from build123d import *

# Parameters (mm, degrees)
ESBO_O1_W                  = 46
ESBO_O1_H                  = 40.25
ESBO_O1_R                  = 14
RESSALTO_EXTRUS_O1_DEPTH   = 5.3
ESBO_O2_W                  = 41.7
ESBO_O2_H                  = 40.25
ESBO_O2_R                  = 1.025
RESSALTO_EXTRUS_O2_DEPTH   = 3
ESBO_O3_W                  = 49
ESBO_O3_H                  = 41.7
RESSALTO_EXTRUS_O3_DEPTH   = 3
ESBO_O4_W                  = 41.7
ESBO_O4_H                  = 43.25
RESSALTO_EXTRUS_O4_DEPTH   = 3
ESBO_O5_W                  = 52
ESBO_O5_H                  = 41.7
RESSALTO_EXTRUS_O5_DEPTH   = 3
CORTE_EXTRUS_O1_DEPTH      = 66.274234005
CORTE_EXTRUS_O1_DEPTH_BACK = 66.274234005
ESBO_O7_R                  = 1.025


with BuildPart() as part:
    # Esboço1 → Ressalto-extrusão1 (new body)
    with BuildSketch(Plane.XY):
        Rectangle(ESBO_O1_W, ESBO_O1_H)
        Circle(ESBO_O1_R, mode=Mode.SUBTRACT)
    extrude(amount=-RESSALTO_EXTRUS_O1_DEPTH)

    # Esboço2 → Ressalto-extrusão2 (add)
    with BuildSketch(Plane.ZY.offset(23)):
        with Locations((15.55, 0)):
            Rectangle(ESBO_O2_W, ESBO_O2_H)
        with Locations((32.6, 17.325)):
            Circle(ESBO_O2_R, mode=Mode.SUBTRACT)
        with Locations((10.6, 17.325)):
            Circle(ESBO_O2_R, mode=Mode.SUBTRACT)
        with Locations(Location((10.6, -17.325, 0), (0, 0, 180))):
            Circle(ESBO_O2_R, mode=Mode.SUBTRACT)
        with Locations(Location((32.6, -17.325, 0), (0, 0, 180))):
            Circle(ESBO_O2_R, mode=Mode.SUBTRACT)
        with Locations((2.8, 11.025)):
            Circle(ESBO_O2_R, mode=Mode.SUBTRACT)
        with Locations(Location((2.8, -11.025, 0), (0, 0, 180))):
            Circle(ESBO_O2_R, mode=Mode.SUBTRACT)
    extrude(amount=RESSALTO_EXTRUS_O2_DEPTH)

    # Esboço3 → Ressalto-extrusão3 (add)
    with BuildSketch(Plane(origin=(0, 20.125, 0), x_dir=(1, 0, 0), z_dir=(0, 1, 0))):
        with Locations((-1.5, -15.55)):
            Rectangle(ESBO_O3_W, ESBO_O3_H)
    extrude(amount=RESSALTO_EXTRUS_O3_DEPTH)

    # Esboço4 → Ressalto-extrusão4 (add)
    with BuildSketch(Plane(origin=(23, 0, 0), x_dir=(0, 0, -1), z_dir=(1, 0, 0))):
        with Locations((-15.55, 1.5)):
            Rectangle(ESBO_O4_W, ESBO_O4_H)
    extrude(amount=RESSALTO_EXTRUS_O4_DEPTH)

    # Esboço5 → Ressalto-extrusão5 (add)
    with BuildSketch(Plane(origin=(0, -20.125, 0), x_dir=(-1, 0, 0), z_dir=(0, -1, 0))):
        with Locations((0, -15.55)):
            Rectangle(ESBO_O5_W, ESBO_O5_H)
    extrude(amount=RESSALTO_EXTRUS_O5_DEPTH)

    # Esboço7 → Corte-extrusão1 (cut, two sides: drawn at the far end of the back side and taken through both)
    with BuildSketch(Plane.ZY.offset(23).offset(-CORTE_EXTRUS_O1_DEPTH_BACK)):
        with Locations((2.8, 11.025)):
            Circle(ESBO_O7_R)
        with Locations((10.6, 17.325)):
            Circle(ESBO_O7_R)
        with Locations((32.6, 17.325)):
            Circle(ESBO_O7_R)
        with Locations(Location((2.8, -11.025, 0), (0, 0, 180))):
            Circle(ESBO_O7_R)
        with Locations(Location((10.6, -17.325, 0), (0, 0, 180))):
            Circle(ESBO_O7_R)
        with Locations(Location((32.6, -17.325, 0), (0, 0, 180))):
            Circle(ESBO_O7_R)
    extrude(amount=CORTE_EXTRUS_O1_DEPTH + CORTE_EXTRUS_O1_DEPTH_BACK, mode=Mode.SUBTRACT)


solid = part.part
Design review of the part built by this model. Coordinates are the model's own, in mm. A direction names the side the tool comes from. Round coordinates to 2 decimals unless told otherwise and drop trailing zeros. Write each loop counter-clockwise with the first axis right and the second up, starting at its lowest first coordinate (ties: lowest second). Pieces come first, ordered by that corner, then holes.
Item 1: Consider section D-D on x = -20. Give the boundary of the cut face in (y, z) (3 decimals).
Item 2: Wall thickness on L1, parallel to Y at x = -24.45, z = 32.6 (3 decimals); L2, parallel to Y at x = -24.5, z = 2.8 (3 decimals); L3, parallel to Y at x = -4.5, z = 26.5 (3 decimals): over which ranges is each line inside the solid? List them lowest first.
Item 3: For faces 4 (the cylindrical face through (-24.479, 10.024, 2.578)), 5 (the flat face through (0, -20.125, 18)), list the 3-axis set-ups (+Z, -Z, +X, -X, +Y, -Y) from which the entire face can be reached by the end or side of a thin tool; tool diameter is ignored.
Item 4: Consider section C-C on x = -7. Give the boundary of the cut face in (y, z) (3 decimals).
Item 5: Consider section B-B on z = 2.8. Give the boundary of the cut face in (x, y) (3 decimals), and give its area (3 significant figures).
Item 6: Consider section A-A on y = 0. Give the boundary of the cut face in (x, z), and give its area (3 significant figures).
Item 7: For pin 1 Ø2 at (x, y) = (7, -14) entering from +Z, flat-tipped, find the tip position at first contact; note if it passes through.
Item 8: Draft analysis for pull direction Y (two halves, no side actions). For faces 1 (the cylindrical face through (-24.479, -17.37, 11.624)), 2 (the flat face through (0, 16, -5.3)), 3 (the flat face through (0, 23.125, 16)), state which applies: released by +Y, released by -Y, zero draft, split by the parting line, or undercut.
Check values:
1. outline: (-23.125, -5.3) - (23.125, -5.3) - (23.125, 36.4) - (20.125, 36.4) - (20.125, 0) - (-20.125, 0) - (-20.125, 36.4) - (-23.125, 36.4) - close
2. L1: y = -23.125 to -18.35, -16.3 to 16.3, 18.35 to 23.125
2. L2: y = -23.125 to -12.05, -10 to 10, 12.05 to 23.125
2. L3: y = -23.125 to -20.125, 20.125 to 23.125
3. face 4: +X, -X
3. face 5: +Z
4. outline: (-23.125, -5.3) - (-12.124, -5.3) - (-12.124, 0) - (-20.125, 0) - (-20.125, 36.4) - (-23.125, 36.4) - close; (12.124, -5.3) - (23.125, -5.3) - (23.125, 36.4) - (20.125, 36.4) - (20.125, 0) - (12.124, 0) - close
5. outline: (-26, -23.125) - (26, -23.125) - (26, -12.05) - (23, -12.05) - (23, -20.125) - (-23, -20.125) - (-23, -12.05) - (-26, -12.05) - close; (-26, -10) - (-23, -10) - (-23, 10) - (-26, 10) - close; (-26, 12.05) - (-23, 12.05) - (-23, 20.125) - (23, 20.125) - (23, 12.05) - (26, 12.05) - (26, 23.125) - (-26, 23.125) - close; (23, -10) - (26, -10) - (26, 10) - (23, 10) - close
5. area: 529 mm2
6. outline: (-26, -5.3) - (-14, -5.3) - (-14, 0) - (-23, 0) - (-23, 36.4) - (-26, 36.4) - close; (14, -5.3) - (26, -5.3) - (26, 36.4) - (23, 36.4) - (23, 0) - (14, 0) - close
6. area: 346 mm2
7. pin 1: stops at z = 0
8. face 1: undercut
8. face 2: zero draft
8. face 3: released by +Y
